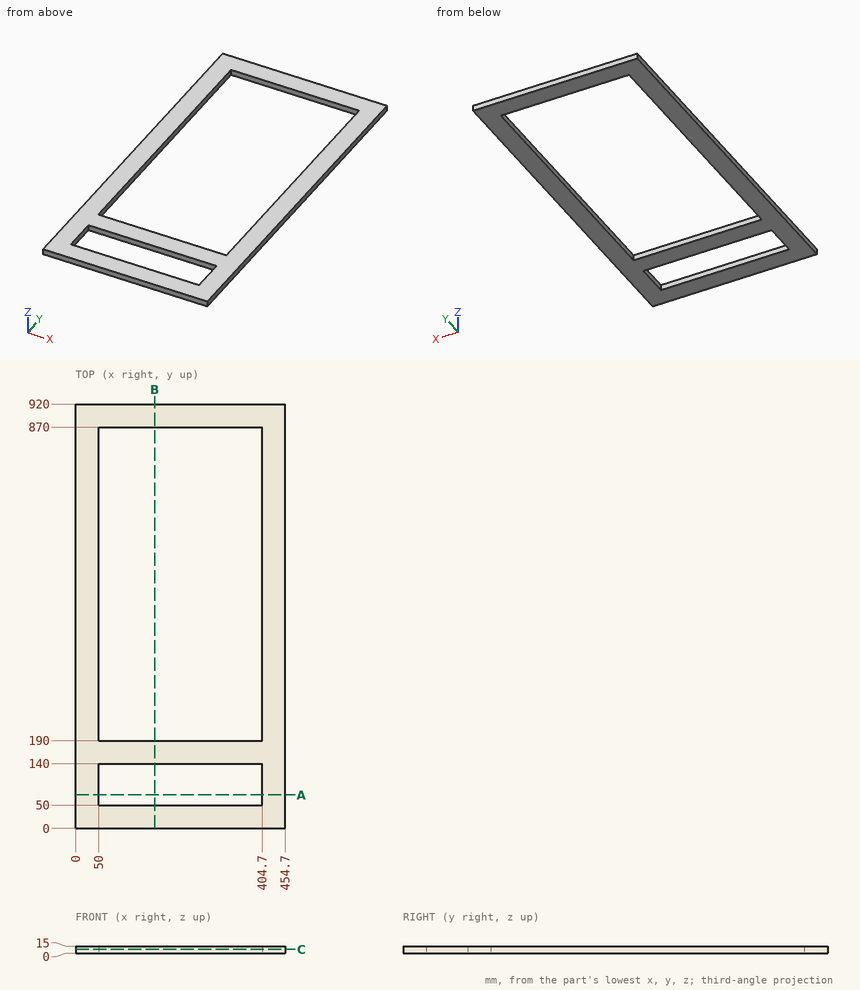
For this review, use the dimensioned drawing (mm, ordinates from the lowest corner) and the shaded views. Round coordinates to 2 decimals unless told otherwise and drop trailing zeros. Order: outer loops, then holes, each group sorted by start corner. A loop starts at its lowest first (then second) coordinate and runs counter-clockwise, first axis right, second up. Notation, with made-up numbers: M 42,5.25 L 62,5.25 A15 ccw 62,20.25 Z; hole C -23,56 d5. An arc over 180 degrees is marked long. Use a Markdown table: item, result.
1) Insertion check: pin 1 (4.5 mm diameter, centred on y = 92.5, z = 11, fed in from -X). The pin has a flat end and moves straight along its axis. Give the tip position at first contact, or say it passes through.
Report:
| item | result |
|---|---|
| pin 1 | x = 0 |
2) Wall thickness on line 1 along Y through (x, z) = (262.5, 5.5); line 2 along X through (y, z) = (766, 2.5): over which ranges is each line inside the solid? List them lowest first. Write a range as [from, to].
Report:
| item | result |
|---|---|
| line 1 | [0, 50], [140, 190], [870, 920] |
| line 2 | [0, 50], [404.7, 454.7] |
3) Consider section C-C (z = 8.5). Write out the cut boundary in (x, y).
Report:
| item | result |
|---|---|
| outline | M 0,0 L 454.7,0 L 454.7,920 L 0,920 Z; hole M 50,50 L 404.7,50 L 404.7,140 L 50,140 Z; hole M 50,190 L 404.7,190 L 404.7,870 L 50,870 Z |
4) Consider section A-A (y = 72.5). Write out the cut boundary in (x, z), then the cut area to 3 significant figures.
Report:
| item | result |
|---|---|
| outline | M 0,0 L 50,0 L 50,15 L 0,15 Z; M 404.7,0 L 454.7,0 L 454.7,15 L 404.7,15 Z |
| area | 1,500 mm^2 |
5) Consider section B-B (x = 171.5). Write out the cut boundary in (y, z), then the cut area to 3 significant figures.
Report:
| item | result |
|---|---|
| outline | M 0,0 L 50,0 L 50,15 L 0,15 Z; M 140,0 L 190,0 L 190,15 L 140,15 Z; M 870,0 L 920,0 L 920,15 L 870,15 Z |
| area | 2,250 mm^2 |
